```python
from build123d import *

# Parameters (mm, degrees)
SKETCH1_W                    = 117.4
SKETCH1_H                    = 39.9
BASE_FLANGE1_DEPTH           = 5
EDGE_FLANGE1_STRIP_W         = 21.4732
EDGE_FLANGE1_STRIP_H         = 5
EDGE_FLANGE1_STRIP_CUT_DEPTH = 39.9
EDGE_FLANGE1_DEPTH           = 39.9
CUT_EXTRUDE1_START           = -5
CUT_EXTRUDE1_DEPTH           = 5


with BuildPart() as part:
    # Base-Flange1: sheet metal written as solids
    # Sketch1 → Base-Flange1 (new body)
    with BuildSketch(Plane.XY):
        Rectangle(SKETCH1_W, SKETCH1_H)
    extrude(amount=-BASE_FLANGE1_DEPTH)

    # Edge-Flange1: sheet metal written as solids
    # Edge-Flange1 strip (on a plane across the edge) → Edge-Flange1 strip cut (cut)
    with BuildSketch(Plane(origin=(58.7, -19.95, 0), x_dir=(-1, 0, 0), z_dir=(0, 1, 0))):
        with Locations((-5, -2.5)):
            Rectangle(EDGE_FLANGE1_STRIP_W, EDGE_FLANGE1_STRIP_H)
    extrude(amount=EDGE_FLANGE1_STRIP_CUT_DEPTH, mode=Mode.SUBTRACT)

    # Edge-Flange1 section (on a plane across the edge) → Edge-Flange1 (add)
    with BuildSketch(Plane(origin=(58.7, -19.95, 0), x_dir=(-1, 0, 0), z_dir=(0, 1, 0))):
        with BuildLine():
            Line((0, 0.7366), (0, 58))
            Line((0, 58), (5, 58))
            Line((5, 58), (5, 0.7366))
            ThreePointArc((5, 0.7366), (5.215745145, 0.215745145), (5.7366, 0))
            Line((5.7366, 0), (5.7366, -5))
            ThreePointArc((5.7366, -5), (1.680211239, -3.319788761), (0, 0.7366))
        make_face()
    extrude(amount=EDGE_FLANGE1_DEPTH)

    # Cut-Extrude1: read off the stored shape, not the designer's step
    # Cut-Extrude1 outline → Cut-Extrude1 (cut)
    with BuildSketch(Plane.XY.offset(CUT_EXTRUDE1_START)):
        with BuildLine():
            ThreePointArc((-38.75, -19.95), (-52.856780317, -14.106780252), (-58.7, 9.1e-08))
            Line((-58.7, 9.1e-08), (-58.7, -19.95))
            Line((-58.7, -19.95), (-38.75, -19.95))
        make_face()
        with BuildLine():
            ThreePointArc((-58.7, 9.1e-08), (-52.856780252, 14.106780317), (-38.75, 19.95))
            Line((-38.75, 19.95), (-58.7, 19.95))
            Line((-58.7, 19.95), (-58.7, 9.1e-08))
        make_face()
        with BuildLine():
            ThreePointArc((42.85, -3.35), (46.2, 0), (42.85, 3.35))
            Line((42.85, 3.35), (-45.35, 3.35))
            ThreePointArc((-45.35, 3.35), (-48.7, 0), (-45.35, -3.35))
            Line((-45.35, -3.35), (42.85, -3.35))
        make_face()
    extrude(amount=CUT_EXTRUDE1_DEPTH, mode=Mode.SUBTRACT)


solid = part.part
```
Geometry check sheet. Reference: the model listing, model coordinates, mm. A direction names the side the tool comes from. Give positions to 0.01 mm unless a question says otherwise; leave off trailing zeros. Loops run counter-clockwise (first coordinate to the right, second up) from the corner with the lowest first, then second, coordinate; pieces in that order, holes last. Notation, with made-up numbers: (19.25, 16.25) - (47.25, 16.25) arc R16 ccw to (47.25, 35.25) - close; hole circle Ø6 at (27.5, -11.5). An arc over 180 degrees is marked (long way). Use CSV: the item, a comma, the result in double quotes. Start each with the question number.
Q1. Section check C-C, the plane z = 42. Record the cut outline in (x, y), and give its area (4 significant figures).
Q2. Access from +Z, -Z, +X, -X, +Y, -Y to the whole of each face (thin tool, end or side, straight path). Record for faces 5 (the face through (-4, 5, 0)), 6 (the face through (-2, -3.35, -3)), 7 (the face through (56, 0, 58)).
Q3. Section check A-A, the plane x = -28. Record the cut outline in (y, z).
Q4. Go/stop test with flat-tipped pins: pin 1 Ø12 at (x, y) = (-4, 3) entering from +Z; pin 2 Ø5 at (x, z) = (-45.5, 2) entering from +Y; pin 3 Ø10 at (y, z) = (-9.5, 6) entering from -X. Record where each tip stops, or that it passes through.
Q5. Section check D-D, the plane y = 13.5. Record the cut outline in (x, z), and give its area (3 significant figures).
Q6. Scan lines: probe 1 along Z at (x, y) = (-39, 7.5); probe 2 along X at (y, z) = (-16.5, 12.5). Record each from-to range of solid material in increasing order. Write a range as from..to.
Q7. Section check B-B, the plane y = -1.5. Record the cut outline in (x, z), and give its area (3 significant figures).
Q8. Release check for a two-part mould opening along Y. For faces 1 (the face through (24, -19.95, -1)), 2 (the face through (24, 19.95, -1)), 3 (the face through (-4, 5, -5)), 4 (the face through (-48.7, 0.1, -2.5)) record: +Y half, -Y half, draft (parallel to the pull), parting line (faces both ways), or undercut.
Findings below:
1,outline,"(53.7, -19.95) - (58.7, -19.95) - (58.7, 19.95) - (53.7, 19.95) - close"
1,area,"199.5 mm^2"
2,face 5,"+Z, -X, +Y, -Y"
2,face 6,"+Z, -Z"
2,face 7,"+Z, +X, -X, +Y, -Y"
3,outline,"(-19.95, -5) - (-3.35, -5) - (-3.35, 0) - (-19.95, 0) - close; (3.35, -5) - (19.95, -5) - (19.95, 0) - (3.35, 0) - close"
4,pin 1,"stops at z = 0"
4,pin 2,"stops at y = 19.25"
4,pin 3,"stops at x = 53.7"
5,outline,"(-53.44, -5) - (52.96, -5) arc R5.74 ccw to (58.7, 0.74) - (58.7, 58) - (53.7, 58) - (53.7, 0.74) arc R0.74 cw to (52.96, 0) - (-53.44, 0) - close"
5,area,"844 mm^2"
6,probe 1,"z = -5..0"
6,probe 2,"x = 53.7..58.7"
7,outline,"(-58.64, -5) - (-48.35, -5) - (-48.35, 0) - (-58.64, 0) - close; (45.85, -5) - (52.96, -5) arc R5.74 ccw to (58.7, 0.74) - (58.7, 58) - (53.7, 58) - (53.7, 0.74) arc R0.74 cw to (52.96, 0) - (45.85, 0) - close"
7,area,"399 mm^2"
8,face 1,"-Y half"
8,face 2,"+Y half"
8,face 3,"draft"
8,face 4,"undercut"
